from build123d import *

# Parameters (mm, degrees)
SKETCH017_W     = 231.34
SKETCH017_H     = 152.71
SKETCH017_W_2   = 217.34
SKETCH017_H_2   = 138.71
PAD009_DEPTH    = 7.5
SKETCH018_W     = 231.34
SKETCH018_H     = 152.71
SKETCH018_W_2   = 84.17
SKETCH018_H_2   = 114.71
PAD010_DEPTH    = 3.5
SKETCH052_R     = 1.5875
POCKET020_DEPTH = 3.5
SKETCH053_R     = 4.44
PAD027_DEPTH    = 2.5


with BuildPart() as part:
    # Sketch017 → Pad009 (new body)
    with BuildSketch(Plane.XY.offset(1.57)):
        with Locations((106.67, 67.355)):
            Rectangle(SKETCH017_W, SKETCH017_H)
        with Locations((106.67, 67.355)):
            Rectangle(SKETCH017_W_2, SKETCH017_H_2, mode=Mode.SUBTRACT)
    extrude(amount=-PAD009_DEPTH)

    # Sketch018 (on Face10 of Pad009) → Pad010 (join)
    with BuildSketch(Plane(origin=(0, 0, -5.93), x_dir=(1, 0, 0), z_dir=(0, 0, -1))):
        with Locations((106.67, -67.355)):
            Rectangle(SKETCH018_W, SKETCH018_H)
        with Locations((52.085, -67.355)):
            Rectangle(SKETCH018_W_2, SKETCH018_H_2, mode=Mode.SUBTRACT)
        with Locations((161.255, -67.355)):
            Rectangle(SKETCH018_W_2, SKETCH018_H_2, mode=Mode.SUBTRACT)
    extrude(amount=PAD010_DEPTH)

    # Sketch052 (on Face13 of Pad010) → Pocket020 (cut)
    with BuildSketch(Plane(origin=(0, 0, -9.43), x_dir=(1, 0, 0), z_dir=(0, 0, -1))):
        with Locations((114.73, -25.365)):
            Circle(SKETCH052_R)
        with Locations((98.61, -55.448259)):
            Circle(SKETCH052_R)
        with Locations((114.73, -78.865)):
            Circle(SKETCH052_R)
        with Locations((98.61, -108.948259)):
            Circle(SKETCH052_R)
    extrude(amount=-POCKET020_DEPTH, mode=Mode.SUBTRACT)

    # Sketch053 (on Face15 of Pocket020) → Pad027 (join)
    with BuildSketch(Plane.XY.offset(-5.93)):
        with Locations((98.61, 108.948259)):
            Circle(SKETCH053_R)
        Polygon((101.56, 107.245076), (101.56, 110.651443), (98.61, 112.354626), (95.66, 110.651443), (95.66, 107.245076), (98.61, 105.541893), align=None, mode=Mode.SUBTRACT)
        with Locations((114.73, 78.865)):
            Circle(SKETCH053_R)
        Polygon((117.68, 77.161817), (117.68, 80.568183), (114.73, 82.271367), (111.78, 80.568183), (111.78, 77.161817), (114.73, 75.458633), align=None, mode=Mode.SUBTRACT)
        with Locations((98.61, 55.448259)):
            Circle(SKETCH053_R)
        Polygon((101.56, 53.745076), (101.56, 57.151443), (98.61, 58.854626), (95.66, 57.151443), (95.66, 53.745076), (98.61, 52.041893), align=None, mode=Mode.SUBTRACT)
        with Locations((114.73, 25.365)):
            Circle(SKETCH053_R)
        Polygon((117.68, 23.661817), (117.68, 27.068183), (114.73, 28.771367), (111.78, 27.068183), (111.78, 23.661817), (114.73, 21.958633), align=None, mode=Mode.SUBTRACT)
    extrude(amount=PAD027_DEPTH)


solid = part.part
Input: part model. Units: mm. Frame: model coordinates. A direction names the side the tool comes from. Coordinates: 2 decimals unless noted, no trailing zeros. Order: outer loops, then holes, each group sorted by start corner. A loop starts at its lowest first (then second) coordinate and runs counter-clockwise, first axis right, second up. Notation, with made-up numbers: M -13.75,-35 L 8.25,-35 A22 ccw 8.25,-9 Z; hole C 88.5,-37.5 d6. An arc over 180 degrees is marked long. One line per question, with ' | ' between items.
Item 1: Pin query (flat end, axial travel): pin 1 (5 mm diameter, centred on x = 114.73, y = 25.365, fed in from +Z); pin 2 (10 mm diameter, centred on x = 115.5, y = 23, fed in from +Z). Return the tip coordinate at first contact, or that it passes through.
Geometry results:
pin 1: stops at z = -5.93 | pin 2: stops at z = -3.43
Item 2: Ray query, line 1 along Y through (x, z) = (98.61, -7.65); line 2 along Y through (x, z) = (114.73, -8.3); line 3 along X through (y, z) = (37.5, -7). Return the intervals inside material, ascending.
Geometry results:
line 1: y = -9 to 53.86, 57.04 to 107.36, 110.54 to 143.71 | line 2: y = -9 to 23.78, 26.95 to 77.28, 80.45 to 143.71 | line 3: x = -9 to 10, 94.17 to 119.17, 203.34 to 222.34
Item 3: Section B-B (y = 100.5). Output: boundary loops of the cut face in (x, z).
Geometry results:
outline: M -9,-9.43 L 10,-9.43 L 10,-5.93 L -2,-5.93 L -2,1.57 L -9,1.57 Z; M 94.17,-9.43 L 119.17,-9.43 L 119.17,-5.93 L 94.17,-5.93 Z; M 203.34,-9.43 L 222.34,-9.43 L 222.34,1.57 L 215.34,1.57 L 215.34,-5.93 L 203.34,-5.93 Z
Item 4: Reachability of faces 4 (the flat face through (105, 66, -9.43)), 5 (the flat face through (97.6, 58.5, -3.43)) from +Z, -Z, +X, -X, +Y, -Y: full face, straight path, thin tool, end or side. Return the list, or none.
Geometry results:
face 4: -Z, +X, -X, +Y, -Y | face 5: +Z
Item 5: Draft query along X for faces 1 (the flat face through (98, -6, 1.57)), 2 (the flat face through (-9, 68, -4)), 3 (the flat face through (114, 22, -3.43)). Return one class per face: released by +X, released by -X, zero draft, split by the parting line, or undercut.
Geometry results:
face 1: zero draft | face 2: released by -X | face 3: undercut
Item 6: Section A-A (x = 66). Output: boundary loops of the cut face in (y, z).
Geometry results:
outline: M -9,-9.43 L 10,-9.43 L 10,-5.93 L -2,-5.93 L -2,1.57 L -9,1.57 Z; M 124.71,-9.43 L 143.71,-9.43 L 143.71,1.57 L 136.71,1.57 L 136.71,-5.93 L 124.71,-5.93 Z
